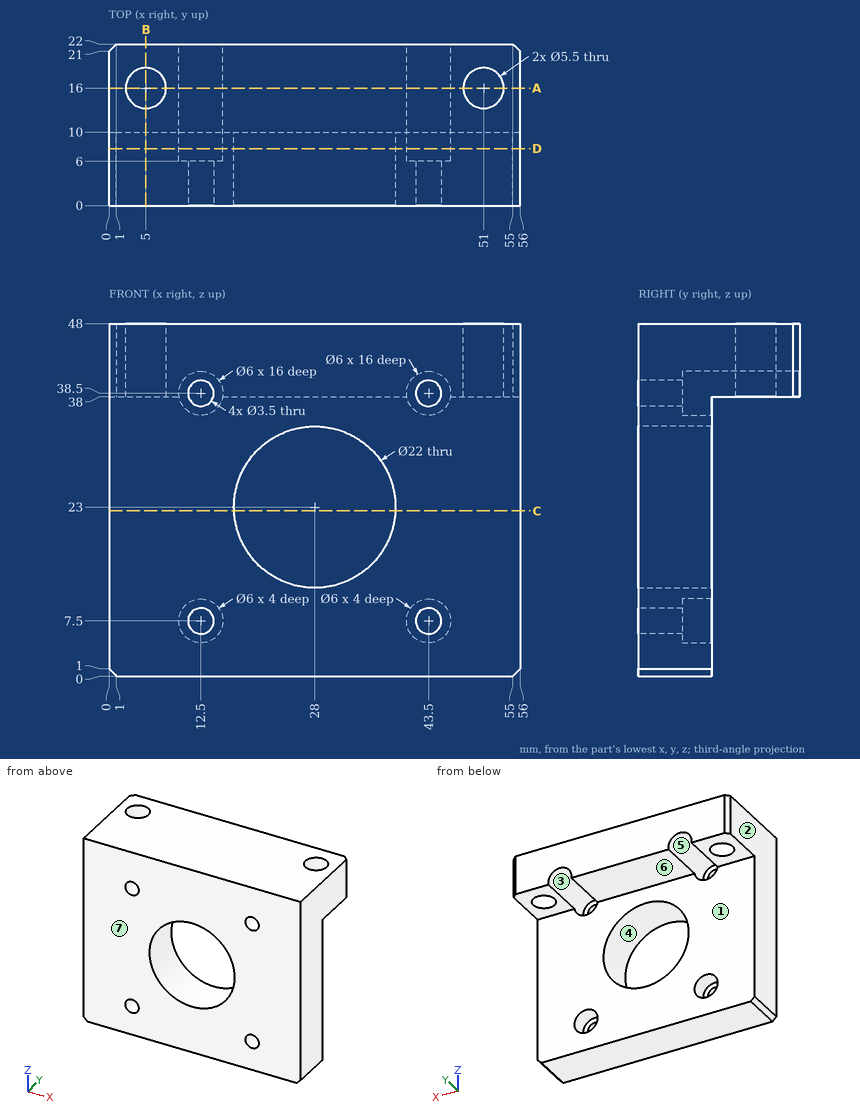
For this review, use the dimensioned drawing (mm, ordinates from the lowest corner) and the shaded views. A direction names the side the tool comes from. Give positions to 0.01 mm unless a question says otherwise; leave off trailing zeros. Loops run counter-clockwise (first coordinate to the right, second up) from the corner with the lowest first, then second, coordinate; pieces in that order, holes last. Notation, with made-up numbers: (-9, 69) -> (17, 69) arc R27 ccw to (17, 86) -> close; hole circle Ø9 at (33, 7). An arc over 180 degrees is marked (long way). One line per question, with ' | ' between items. Start each with the question number.
(1) We need section A-A (y = 16). State the section outline as (x, z) points, and give its area (3 significant figures).
(2) We need section B-B (x = 5). State the section outline as (y, z) points, and give its area (3 significant figures).
(3) We need section C-C (z = 22.5). State the section outline as (x, y) points, and give its area (3 significant figures).
(4) For line 1 (X direction, y = 2.3, z = 7.5); line 2 (X direction, y = 7, z = 7.5); line 3 (Z direction, x = 43.5, y = 1.7), list the stretches that pass through material, from the lowest coordinate up.
(5) Insertion check: P1, Ø9, axis at x = 5, y = 16, coming from the -Z side; P2, Ø3, axis at x = 45, z = 37, coming from the +Y side; P3, Ø3, axis at x = 13.5, z = 39.5, coming from the +Y side. Each pin has a flat end and moves straight along its axis. Give the tip position at first contact, or say it passes through.
(6) For the marked faces 5, 6 and 7, list the 3-axis set-ups (+Z, -Z, +X, -X, +Y, -Y) from which the entire face can be reached by the end or side of a thin tool; tool diameter is ignored.
(7) Draft analysis for pull direction X (two halves, no side actions). For the marked faces 1, 2, 3 and 4, state which applies: +X half, -X half, draft (parallel to the pull), parting line (faces both ways), or undercut.
(8) We need section D-D (y = 7.75). State the section outline as (x, z) points.
The answers:
1) outline: (0, 38) -> (2.25, 38) -> (2.25, 48) -> (0, 48) -> close; (7.75, 38) -> (9.54, 38) arc R3 cw (long way) to (15.46, 38) -> (40.54, 38) arc R3 cw (long way) to (46.46, 38) -> (48.25, 38) -> (48.25, 48) -> (7.75, 48) -> close; (53.75, 38) -> (56, 38) -> (56, 48) -> (53.75, 48) -> close | area: 416 mm^2
2) outline: (0, 0) -> (10, 0) -> (10, 38) -> (13.25, 38) -> (13.25, 48) -> (0, 48) -> close; (18.75, 38) -> (22, 38) -> (22, 48) -> (18.75, 48) -> close | area: 545 mm^2
3) outline: (0, 0) -> (17.01, 0) -> (17.01, 10) -> (0, 10) -> close; (38.99, 0) -> (56, 0) -> (56, 10) -> (38.99, 10) -> close | area: 340 mm^2
4) line 1: x = 0 to 10.75, 14.25 to 41.75, 45.25 to 56 | line 2: x = 0 to 9.5, 15.5 to 40.5, 46.5 to 56 | line 3: z = 0 to 5.75, 9.25 to 36.75, 40.25 to 48
5) P1: stops at z = 38 | P2: stops at y = 10 | P3: stops at y = 6
6) face 5: +Y | face 6: -Z, +X, -X, +Y | face 7: +Z, -Z, +X, -X, -Y
7) face 1: draft | face 2: -X half | face 3: undercut | face 4: undercut
8) outline: (0, 1) -> (1, 0) -> (55, 0) -> (56, 1) -> (56, 48) -> (0, 48) -> close; hole circle Ø6 at (12.5, 7.5); hole circle Ø6 at (12.5, 38.5); hole circle Ø22 at (28, 23); hole circle Ø6 at (43.5, 7.5); hole circle Ø6 at (43.5, 38.5)
